```python
from build123d import *

# Parameters (mm, degrees)
SKETCH14_W = 8.1026
SKETCH14_H = 257.175


with BuildPart() as part:
    # Sketch3 → Revolve1 (revolve)
    with BuildSketch(Plane.XY, mode=Mode.PRIVATE) as revolve1_sk:
        Polygon((0, -1184.275), (0, -1216.025), (13.3985, -1216.025), (12.08405, -1184.275), align=None)
    revolve(revolve1_sk.sketch.rotate(Axis((0, -1184.275, 0), (0, -1, 0)), 180), axis=Axis((0, -1184.275, 0), (0, -1, 0)))



with BuildPart() as body_2:
    # Sketch1 → Revolve3 (revolve)
    with BuildSketch(Plane.XY, mode=Mode.PRIVATE) as revolve3_sk:
        Polygon((0, 0), (11.354913135, 0), (9.947052362, -168.275), (0, -168.275), align=None)
    revolve(revolve3_sk.sketch.rotate(Axis((0, 0, 0), (0, -1, 0)), 180), axis=Axis((0, 0, 0), (0, -1, 0)))

    # Sketch8 → Revolve4 (revolve)
    with BuildSketch(Plane.XY, mode=Mode.PRIVATE) as revolve4_sk:
        Polygon((0, -168.275), (0, -320.675), (0, -330.2), (9.144, -330.2), (8.07085, -320.675), (8.07085, -168.275), align=None)
    revolve(revolve4_sk.sketch.rotate(Axis((0, -168.275, 0), (0, -1, 0)), 180), axis=Axis((0, -168.275, 0), (0, -1, 0)))

    # Sketch11 → Revolve5 (revolve)
    with BuildSketch(Plane.XY, mode=Mode.PRIVATE) as revolve5_sk:
        Polygon((0, -330.2), (0, -619.125), (0, -628.65), (9.144, -628.65), (8.0645, -619.125), (8.0645, -330.2), align=None)
    revolve(revolve5_sk.sketch.rotate(Axis((0, -330.2, 0), (0, -1, 0)), 180), axis=Axis((0, -330.2, 0), (0, -1, 0)))

    # Sketch13 → Revolve6 (revolve)
    with BuildSketch(Plane.XY, mode=Mode.PRIVATE) as revolve6_sk:
        Polygon((0, -628.65), (8.04545, -628.65), (8.04545, -917.575), (9.144, -927.1), (0, -927.1), align=None)
    revolve(revolve6_sk.sketch.rotate(Axis((0, -628.65, 0), (0, -1, 0)), 180), axis=Axis((0, -628.65, 0), (0, -1, 0)))


with BuildPart() as part_1:
    add(part.part)

    add(body_2.part)  # Revolve7 merges body 2
    # Sketch14 → Revolve7 (revolve)
    with BuildSketch(Plane.XY, mode=Mode.PRIVATE) as revolve7_sk:
        with Locations((4.0513, -1055.6875)):
            Rectangle(SKETCH14_W, SKETCH14_H)
    revolve(revolve7_sk.sketch.rotate(Axis((0, -927.1, 0), (0, -1, 0)), 180), axis=Axis((0, -927.1, 0), (0, -1, 0)))


solid = part_1.part
```
Geometry check sheet. Reference: the model listing, model coordinates, mm. A direction names the side the tool comes from. Give positions to 0.01 mm unless a question says otherwise; leave off trailing zeros. Order: outer loops, then holes, each group sorted by start corner. A loop starts at its lowest first (then second) coordinate and runs counter-clockwise, first axis right, second up. Notation, with made-up numbers: (47.25, -13.75) - (104.25, -13.75) arc R31 ccw to (104.25, 23.25) - close; hole circle Ø11 at (-11.75, 29). An arc over 180 degrees is marked (long way). Answer in a Markdown table with one row per item. Add a question column.
Q1. Gauge pin test, flat ends, axial feed: pin 1 (5 mm diameter, centred on y = -233.5, z = -4.5, fed in from +X); pin 2 (12 mm diameter, centred on y = -1040.5, z = 1.5, fed in from -X); pin 3 (6 mm diameter, centred on x = 6, y = -982.5, fed in from +Z). Record the tip position at first contact, or that the pin passes through.
Q2. Tool access check on faces 4 (the flat face through (0, 0, 0)), 5 (the conical face through (1.838, -622.762, 8.275)). Record the directions out of +Z, -Z, +X, -X, +Y, -Y that give a thin tool (end or side, any length) a straight path to the whole face; none if there is none.
Q3. Cross-section at A-A, the plane y = -577. Enter the section's corners in (x, z), then the cut area to 3 significant figures.
Q4. Mould release check, pull along Y, two halves, no side actions. Record for faces 1 (the conical face through (-12.144, -1199.928, -3.824)), 2 (the flat face through (0.8, -168.275, -8.2)), 3 (the flat face through (0, -1216.025, 0)): pulls with the +Y half, pulls with the -Y half, needs draft (parallel to the pull), parting line crosses it, or undercut.
Q5. Material ranges on probe 1 along Y at (x, z) = (-2.75, 9.5) (3 decimals); probe 2 along Z at (x, y) = (1.5, -260.5); probe 3 along Y at (x, z) = (-5.5, -10) (3 decimals), recorded low to high. Write a range as from..to.
Q6. Cross-section at B-B, the plane y = -969.5. Enter the section's corners in (x, z), then the cut area to 3 significant figures.
Check values:
| question | item | result |
|---|---|---|
| 1 | pin 1 | stops at x = 7.82 |
| 1 | pin 2 | stops at x = -8.1 |
| 1 | pin 3 | stops at z = 7.53 |
| 2 | face 4 | +Z, -Z, +X, -X, +Y |
| 2 | face 5 | none |
| 3 | outline | circle Ø16.13 at (0, 0) |
| 3 | area | 204 mm^2 |
| 4 | face 1 | pulls with the +Y half |
| 4 | face 2 | undercut |
| 4 | face 3 | pulls with the -Y half |
| 5 | probe 1 | y = -1216.025..-1184.275, -168.275..0 |
| 5 | probe 2 | z = -7.93..7.93 |
| 5 | probe 3 | y = -1216.025..-1184.275 |
| 6 | outline | circle Ø16.21 at (0, 0) |
| 6 | area | 206 mm^2 |
